Can you work these out from the model? Positions are in its coordinate system, mm. A direction names the side the tool comes from. Give positions to 0.01 mm unless a question says otherwise; leave off trailing zeros. Write each loop counter-clockwise with the first axis right and the second up, starting at its lowest first coordinate (ties: lowest second). Pieces come first, ordered by that corner, then holes.
from build123d import *

# Parameters (mm, degrees)
SKETCH1_W           = 0.8
SKETCH1_H           = 219.088379857
BOSS_EXTRUDE2_DEPTH = 4
BOSS_EXTRUDE3_DEPTH = 3.575


with BuildPart() as part:
    # Sketch1 → Revolve1 (revolve)
    with BuildSketch(Plane.XY, mode=Mode.PRIVATE) as revolve1_sk:
        with Locations((3.575, -190.824189929)):
            Rectangle(SKETCH1_W, SKETCH1_H)
    revolve(revolve1_sk.sketch.rotate(Axis((0, 0, 0), (0, -1, 0)), 180), axis=Axis((0, 0, 0), (0, -1, 0)))

    # Sketch17 → Boss-Extrude2 (add)
    with BuildSketch(Plane(origin=(0, 58.900156663, 0), x_dir=(1, 0, 0), z_dir=(0, 0, 1))):
        with BuildLine():
            ThreePointArc((6.5, -160.693323683), (0, -158.680156663), (-6.5, -160.693323683))
            Line((-6.5, -160.693323683), (-6.5, -179.666989644))
            ThreePointArc((-6.5, -179.666989644), (0, -181.680156663), (6.5, -179.666989644))
            Line((6.5, -179.666989644), (6.5, -160.693323683))
        make_face()
        with BuildLine():
            Line((-6.5, -179.666989644), (-6.5, -160.693323683))
            ThreePointArc((-6.5, -160.693323683), (-11.5, -170.180156663), (-6.5, -179.666989644))
        make_face()
        with BuildLine():
            Line((6.5, -156.180156663), (-6.5, -156.180156663))
            Line((-6.5, -156.180156663), (-6.5, -160.693323683))
            ThreePointArc((-6.5, -160.693323683), (0, -158.680156663), (6.5, -160.693323683))
            Line((6.5, -160.693323683), (6.5, -156.180156663))
        make_face()
        with BuildLine():
            ThreePointArc((11.5, -170.180156663), (10.173494975, -164.818254016), (6.5, -160.693323683))
            Line((6.5, -160.693323683), (6.5, -179.666989644))
            ThreePointArc((6.5, -179.666989644), (10.173494975, -175.542059311), (11.5, -170.180156663))
        make_face()
        with BuildLine():
            ThreePointArc((6.5, -179.666989644), (0, -181.680156663), (-6.5, -179.666989644))
            Line((-6.5, -179.666989644), (-6.5, -184.180156663))
            Line((-6.5, -184.180156663), (6.5, -184.180156663))
            Line((6.5, -184.180156663), (6.5, -179.666989644))
        make_face()
    extrude(amount=BOSS_EXTRUDE2_DEPTH)

    # Sketch18 → Boss-Extrude3 (add)
    with BuildSketch(Plane.XY.offset(4)):
        with BuildLine():
            ThreePointArc((-6.5, -101.793167019), (-11.5, -111.28), (-6.5, -120.766832981))
            Line((-6.5, -120.766832981), (-6.5, -119.779411744))
            ThreePointArc((-6.5, -119.779411744), (-10.7, -111.28), (-6.5, -102.780588256))
            Line((-6.5, -102.780588256), (-6.5, -101.793167019))
        make_face()
        with BuildLine():
            Line((6.5, -119.779411744), (6.5, -120.766832981))
            ThreePointArc((6.5, -120.766832981), (10.173494975, -116.641902647), (11.5, -111.28))
            ThreePointArc((11.5, -111.28), (10.173494975, -105.918097353), (6.5, -101.793167019))
            Line((6.5, -101.793167019), (6.5, -102.780588256))
            ThreePointArc((6.5, -102.780588256), (9.592705562, -106.539746842), (10.7, -111.28))
            ThreePointArc((10.7, -111.28), (9.592705562, -116.020253158), (6.5, -119.779411744))
        make_face()
    extrude(amount=BOSS_EXTRUDE3_DEPTH)


solid = part.part
(1) Imagine slicing it at A-A, the plane x = 0. Write out the boundary of the cut face in (y, z) (3 decimals).
Returned:
outline: (-300.368, -3.975) - (-81.28, -3.975) - (-81.28, -3.175) - (-300.368, -3.175) - close; (-300.368, 3.175) - (-125.28, 3.175) - (-125.28, 0) - (-97.28, 0) - (-97.28, 3.175) - (-81.28, 3.175) - (-81.28, 3.975) - (-97.28, 3.975) - (-97.28, 4) - (-125.28, 4) - (-125.28, 3.975) - (-300.368, 3.975) - close
(2) If I drill on L1, parallel to Z at x = 0, y = -206 (3 decimals); L2, parallel to X at y = -251, z = 0.5; L3, parallel to Y at x = -2, z = 1.5, over which ranges is the centre line in solid material (lowest first)?
Returned:
L1: z = -3.975 to -3.175, 3.175 to 3.975
L2: x = -3.94 to -3.14, 3.14 to 3.94
L3: y = -125.28 to -97.28
(3) If we mould it in two halves opening along Y, with no side actions, what happens to faces 6 (the face through (0.41, -189.29, -3.15)), 7 (the face through (0, -111, 4)), 8 (the face through (-3, -81.28, 2))? For each: +Y half, -Y half, draft (parallel to the pull), parting line (faces both ways), or undercut.
Returned:
face 6: draft
face 7: undercut
face 8: +Y half
(4) For faces 1 (the face through (-7, -111, 0)), 2 (the face through (-3, -125.28, 3)), 3 (the face through (6.5, -123, 2)), 4 (the face through (7, -111, 0)), 5 (the face through (0, -111, 0)), which set-ups out of +Z, -Z, +X, -X, +Y, -Y let a thin tool reach every point of the face, with its end or its side?
Returned:
face 1: -Z, -X, +Y, -Y
face 2: +Z, -Y
face 3: +Z, -Z, +X, -Y
face 4: -Z, +X, +Y, -Y
face 5: +Y, -Y
(5) Imagine slicing it at B-B, the plane y = -246. Write out the boundary of the cut face in (x, z) (3 decimals), plus the area to 3 significant figures.
Returned:
outline: circle Ø7.95 at (0, 0); hole circle Ø6.35 at (0, 0)
area: 18.0 mm2
(6) Will these pins go through, and if not, where does the flat tip stop? P1, Ø2, axis at x = -1.5, z = 2, coming from the +Y side; P2, Ø6, axis at x = -7, z = 5.5, coming from the -Y side; P3, Ø10, axis at x = -7, y = -239.5, coming from the -Z side; P4, Ø3, axis at y = -123, z = 2.5, coming from the -X side.
Returned:
P1: stops at y = -81.28
P2: stops at y = -125.28
P3: stops at z = -3.44
P4: stops at x = -6.5
